```python
from build123d import *

# Parameters (mm, degrees)
SCALE_1_SCALE = 2.2


with BuildPart() as part:
    # Эскиз1 → Повернуть1 (revolve)
    with BuildSketch(Plane.XY, mode=Mode.PRIVATE) as revolve_1_sk:
        Polygon((0, 0), (0, 11), (-2.5, 11), (-2.5, 10), (-1.5, 10), (-1.5, 1), (-2.5, 1), (-2.5, 0), align=None)
    revolve(revolve_1_sk.sketch.rotate(Axis((0, 0, 0), (0, 1, 0)), 270), axis=Axis((0, 0, 0), (0, 1, 0)))


with BuildPart() as part_1:
    # Масштаб1: scaled about (0, 5.5, 0)
    add(part.part.scale(SCALE_1_SCALE).moved(Location((0, -6.6, 0))))


solid = part_1.part
```
The model under review builds one solid part; all positions refer to its coordinate system, in mm. A direction names the side the tool comes from. Round coordinates to 2 decimals unless told otherwise and drop trailing zeros. Write each loop counter-clockwise with the first axis right and the second up, starting at its lowest first coordinate (ties: lowest second). Pieces come first, ordered by that corner, then holes. Notation, with made-up numbers: (-25, 12.5) -> (19, 12.5) arc R5 cw to (19, 20.5) -> close; hole circle Ø7 at (0, 44.25). An arc over 180 degrees is marked (long way). Use CSV: the item, a comma, the result in double quotes.
Q1. To check wall thickness, follow probe 1 along Y at (x, z) = (2.75, -4.25); probe 2 along X at (y, z) = (13, 1.25); probe 3 along Z at (x, y) = (-3, -1.25). State the ranges of each line that lie inside material, in increasing order. Write a range as [from, to].
Checks:
probe 1,"[-6.6, -4.4], [15.4, 17.6]"
probe 2,"[-3.05, 3.05]"
probe 3,"[-1.37, 1.37]"
Q2. For pin 1 Ø5 at (x, y) = (-3, 12.5) entering from -Z; pin 2 Ø4 at (x, y) = (-4, 4.5) entering from +Z; pin 3 Ø2 at (x, y) = (2.5, 11) entering from +Z, all flat-tipped, find the tip position at first contact; note any pin that passes through.
Checks:
pin 1,"z = -3.26"
pin 2,"z = 2.62"
pin 3,"z = 2.94"
Q3. Consider section C-C (z = 0). Give the boundary of the cut face in (x, y), then the cut area to 3 significant figures.
Checks:
outline,"(-5.5, -6.6) -> (5.5, -6.6) -> (5.5, -4.4) -> (3.3, -4.4) -> (3.3, 15.4) -> (5.5, 15.4) -> (5.5, 17.6) -> (-5.5, 17.6) -> (-5.5, 15.4) -> (-3.3, 15.4) -> (-3.3, -4.4) -> (-5.5, -4.4) -> close"
area,"179 mm²"
Q4. Consider section D-D (x = 0). Give the boundary of the cut face in (y, z), then the cut area to 3 significant figures.
Checks:
outline,"(-6.6, -5.5) -> (-4.4, -5.5) -> (-4.4, -3.3) -> (15.4, -3.3) -> (15.4, -5.5) -> (17.6, -5.5) -> (17.6, 5.5) -> (15.4, 5.5) -> (15.4, 3.3) -> (-4.4, 3.3) -> (-4.4, 5.5) -> (-6.6, 5.5) -> close"
area,"179 mm²"
Q5. Mouldability with a two-part tool opening along Y and no side actions: class faces 3 (the cylindrical face through (-0.1, 5.4, 3.3)), 4 (the flat face through (0, 17.6, 0)), 5 (the cylindrical face through (5.37, 16.48, 1.19)) as released by +Y, released by -Y, zero draft, split by the parting line, or undercut.
Checks:
face 3,"undercut"
face 4,"released by +Y"
face 5,"zero draft"
Q6. Consider section A-A (z = 4). Give the boundary of the cut face in (x, y), then the cut area to 3 significant figures.
Checks:
outline,"(-3.77, -6.6) -> (3.77, -6.6) -> (3.77, -4.4) -> (-3.77, -4.4) -> close; (-3.77, 15.4) -> (3.77, 15.4) -> (3.77, 17.6) -> (-3.77, 17.6) -> close"
area,"33.2 mm²"
Q7. Consider section B-B (x = 4). Give the boundary of the cut face in (y, z).
Checks:
outline,"(-6.6, -3.77) -> (-4.4, -3.77) -> (-4.4, 3.77) -> (-6.6, 3.77) -> close; (15.4, -3.77) -> (17.6, -3.77) -> (17.6, 3.77) -> (15.4, 3.77) -> close"
Q8. For faces 1 (the flat face through (0, 15.4, -4)), 2 (the flat face through (0, -6.6, 0)), list the 3-axis set-ups (+Z, -Z, +X, -X, +Y, -Y) from which the entire face can be reached by the end or side of a thin tool; tool diameter is ignored.
Checks:
face 1,"none"
face 2,"+Z, -Z, +X, -X, -Y"
